Design review of the part built by this model. Coordinates are the model's own, in mm. Face numbers are marked on the shaded views. A direction names the side the tool comes from. Coordinates: 2 decimals unless noted, no trailing zeros. Write each loop counter-clockwise with the first axis right and the second up, starting at its lowest first coordinate (ties: lowest second). Pieces come first, ordered by that corner, then holes. Notation, with made-up numbers: (75.5, -14.75) -> (114.5, -14.75) arc R21 ccw to (114.5, -1.75) -> close; hole circle Ø9 at (67.25, 80.25). An arc over 180 degrees is marked (long way). Answer in a Markdown table with one row per item. Add a question column.
Item 1: Take a section at B-B, the plane z = 0. Write out the cut boundary in (x, y).
Item 2: Draft analysis for pull direction X (two halves, no side actions). For the marked faces 4, 5 and 6, state which applies: released by +X, released by -X, zero draft, split by the parting line, or undercut.
Item 3: Take a section at A-A, the plane y = 6. Write out the cut boundary in (x, z), and give its area (3 significant figures).
Item 4: To check wall thickness, follow line 1 (X direction, y = 5.75, z = 1.5); line 2 (X direction, y = 1, z = -2); line 3 (Y direction, x = 7.25, z = 3). State the ranges of each line that lie inside material, in increasing order.
Item 5: For the marked faces 1, 2 and 3, list the 3-axis set-ups (+Z, -Z, +X, -X, +Y, -Y) from which the entire face can be reached by the end or side of a thin tool; tool diameter is ignored.
Item 6: Clearance check with flat-ended pins moving along their axes: P1, Ø1.7, axis at y = 5, z = 0.5, coming from the +X side; P2, Ø1.7, axis at x = -2, z = 0, coming from the +Y side; P3, Ø2.5, axis at x = 10.795, z = 0, coming from the +Y side; P4, Ø1, axis at y = 4.5, z = 2.5, coming from the +X side. State where each tip first meets the part, or that it passes through.
Item 7: Take a section at D-D, the plane y = 4. Write out the cut boundary in (x, z), and give its area (3 significant figures).
Item 8: Take a section at C-C, the plane x = -4.75. Write out the cut boundary in (y, z) (3 decimals).
from build123d import *

# Parameters (mm, degrees)
SKETCH1_W           = 25.4
SKETCH1_H           = 8.89
BOSS_EXTRUDE1_DEPTH = 2.54
SKETCH2_W           = 17.018
SKETCH2_H           = 3.302
BOSS_EXTRUDE2_DEPTH = 2.032
SKETCH3_R           = 1.0414
CUT_EXTRUDE1_DEPTH  = 5.572
SKETCH4_W           = 3.302
SKETCH4_H           = 3.302
CUT_EXTRUDE2_DEPTH  = 4.572
SKETCH5_W           = 2.032
SKETCH5_H           = 3.302
BOSS_EXTRUDE3_DEPTH = 2.286
FILLET1_R           = 2.54
FILLET2_R           = 0.508


with BuildPart() as part:
    # Sketch1 → Boss-Extrude1 (new body)
    with BuildSketch(Plane(origin=(0, 0, 0), x_dir=(1, 0, 0), z_dir=(0, 1, 0))):
        Rectangle(SKETCH1_W, SKETCH1_H)
    extrude(amount=BOSS_EXTRUDE1_DEPTH)

    # Sketch2 → Boss-Extrude2 (add)
    with BuildSketch(Plane(origin=(0, 2.54, 0), x_dir=(1, 0, 0), z_dir=(0, 1, 0))):
        with Locations((-0.381, 0)):
            Rectangle(SKETCH2_W, SKETCH2_H)
    extrude(amount=BOSS_EXTRUDE2_DEPTH)

    # Sketch3 → Cut-Extrude1 (cut, through all)
    with BuildSketch(Plane.XZ):
        with Locations((-10.795, 0)):
            Circle(SKETCH3_R)
        with Locations((10.795, 0)):
            Circle(SKETCH3_R)
    extrude(amount=-CUT_EXTRUDE1_DEPTH, mode=Mode.SUBTRACT)

    # Sketch4 → Cut-Extrude2 (cut)
    with BuildSketch(Plane(origin=(0, 4.572, 0), x_dir=(1, 0, 0), z_dir=(0, 1, 0))):
        with Locations((-7.239, 0)):
            Rectangle(SKETCH4_W, SKETCH4_H)
    extrude(amount=-CUT_EXTRUDE2_DEPTH, mode=Mode.SUBTRACT)

    # Sketch5 → Boss-Extrude3 (add)
    with BuildSketch(Plane(origin=(0, 4.572, 0), x_dir=(1, 0, 0), z_dir=(0, 1, 0))):
        with Locations((-4.572, 0)):
            Rectangle(SKETCH5_W, SKETCH5_H)
        with Locations((1.27, 0)):
            Rectangle(SKETCH5_W, SKETCH5_H)
        with Locations((7.112, 0)):
            Rectangle(SKETCH5_W, SKETCH5_H)
    extrude(amount=BOSS_EXTRUDE3_DEPTH)

    # Fillet1
    fillet1_edges = [part.edges().sort_by_distance(p)[0] for p in [
        (12.7, 1.27, 4.445),
        (-12.7, 1.27, 4.445),
        (-12.7, 1.27, -4.445),
        (12.7, 1.27, -4.445),
    ]]
    fillet(fillet1_edges, radius=FILLET1_R)

    # Fillet2
    fillet2_edges = [part.edges().sort_by_distance(p)[0] for p in [
        (12.7, 0, 0),
        (0, 0, 4.445),
        (-12.7, 0, 0),
        (0, 0, -4.445),
        (-11.956051224, 0, -3.701051224),
        (-11.956051224, 0, 3.701051224),
        (11.956051224, 0, -3.701051224),
        (11.956051224, 0, 3.701051224),
    ]]
    fillet(fillet2_edges, radius=FILLET2_R)


solid = part.part
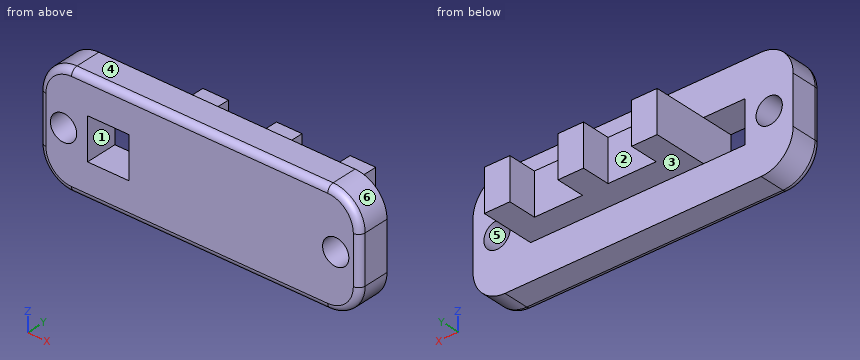
Answers:
| question | item | result |
|---|---|---|
| 1 | outline | (-12.7, 0.51) arc R0.51 ccw to (-12.19, 0) -> (-11.84, 0) -> (-11.84, 2.54) -> (-12.7, 2.54) -> close; (-9.75, 0) -> (-8.89, 0) -> (-8.89, 2.54) -> (-9.75, 2.54) -> close; (-5.59, 0) -> (9.75, 0) -> (9.75, 2.54) -> (8.13, 2.54) -> (8.13, 6.86) -> (6.1, 6.86) -> (6.1, 4.57) -> (2.29, 4.57) -> (2.29, 6.86) -> (0.25, 6.86) -> (0.25, 4.57) -> (-3.56, 4.57) -> (-3.56, 6.86) -> (-5.59, 6.86) -> close; (11.84, 0) -> (12.19, 0) arc R0.51 ccw to (12.7, 0.51) -> (12.7, 2.54) -> (11.84, 2.54) -> close |
| 2 | face 4 | zero draft |
| 2 | face 5 | undercut |
| 2 | face 6 | released by +X |
| 3 | outline | (-5.59, -1.65) -> (-3.56, -1.65) -> (-3.56, 1.65) -> (-5.59, 1.65) -> close; (0.25, -1.65) -> (2.29, -1.65) -> (2.29, 1.65) -> (0.25, 1.65) -> close; (6.1, -1.65) -> (8.13, -1.65) -> (8.13, 1.65) -> (6.1, 1.65) -> close |
| 3 | area | 20.1 mm^2 |
| 4 | line 1 | x = -5.59 to -3.56, 0.25 to 2.29, 6.1 to 8.13 |
| 4 | line 2 | x = -12.7 to 12.7 |
| 4 | line 3 | y = 0 to 2.54 |
| 5 | face 1 | +Y, -Y |
| 5 | face 2 | +Z, -Z, +Y |
| 5 | face 3 | -Z, +X, -X, +Y |
| 6 | P1 | stops at x = 8.13 |
| 6 | P2 | stops at y = 4.57 |
| 6 | P3 | stops at y = 2.54 |
| 6 | P4 | passes through |
| 7 | outline | (-5.59, -1.65) -> (8.13, -1.65) -> (8.13, 1.65) -> (-5.59, 1.65) -> close |
| 7 | area | 45.3 mm^2 |
| 8 | outline | (0, -3.937) arc R0.508 ccw to (0.508, -4.445) -> (2.54, -4.445) -> (2.54, -1.651) -> (6.858, -1.651) -> (6.858, 1.651) -> (2.54, 1.651) -> (2.54, 4.445) -> (0.508, 4.445) arc R0.508 ccw to (0, 3.937) -> close |
